Autodesk Inventor part; units mm, degrees
ref_plane "YZ Plane" through (0, 0, 0) normal (1, 0, 0) x (0, 1, 0)
ref_plane "XZ Plane" through (0, 0, 0) normal (0, 1, 0) x (-1, 0, 0)
ref_plane "XY Plane" through (0, 0, 0) normal (0, 0, 1) x (1, 0, 0)
sketch "Sketch2" plane through (0, 0, 0) normal (0, 1, 0) x (-1, 0, 0)
  line L0 (8.7236, 13.4517) -> (-1.2764, 13.4517)
  line L1 (-1.2764, 13.4517) -> (-1.2764, -3.0483)
  line L2 (-1.2764, -3.0483) -> (8.7236, -3.0483)
  line L3 (8.7236, -3.0483) -> (8.7236, 13.4517)
  point P0 (0, 0)
  dimension "d2" = 10
  dimension "d3" = 16.5
extrude "Extrusion1" add sketch "Sketch2" along normal blind 3
ref_plane "Work Plane1" through (-8.7236, 0, 6.9517) normal (0, 0, 1) x (1, 0, 0)
sketch "Sketch5" plane through (-8.7236, 0, 13.4517) normal (0, 0, 1) x (1, 0, 0)
  line L0 (0, 3) -> (10, 3)
  line L1 (-3, 0) -> (3, 0)
  line L2 (3, 0) -> (3, 6)
  line L3 (3, 6) -> (-3, 6)
  line L4 (-3, 6) -> (-3, 0)
  line L5 (0, 0) -> (10, 0)
  point P0 (8.7236, 0)
  dimension "d41" = 6
  dimension "d42" = 6
  dimension "d43" = 3
extrude "Extrusion4" cut sketch "Sketch5" against normal blind 6.5
sketch "Sketch6" plane through (-8.7236, 0, 6.9517) normal (0, 0, 1) x (1, 0, 0)
  circle A0 centre (0, 3) radius 3
  arc A1 (0, 0) -> (3, 3) centre (0, 3) ccw
  point P0 (8.7236, 0)
  point P1 (0, 0.5)
  dimension "d16" = 6
extrude "Extrusion5" add sketch "Sketch6" against normal blind 5
sketch "Sketch7" plane through (-8.7236, 0, 6.9517) normal (0, 0, 1) x (1, 0, 0)
  arc A0 (3, 3) -> (0, 0) centre (0, 3) ccw
  circle A1 centre (0, 3) radius 1.75
  line L0 (3, 0) -> (0, 0)
  line L1 (3, 3) -> (3, 0)
  point P0 (8.7236, 0)
  dimension "d20" = 3.5
extrude "Extrusion6" cut sketch "Sketch7" against normal up to next contours A1
sketch "Sketch9" plane through (0, 3, 0) normal (0, 1, 0) x (1, 0, 0)
  circle A0 centre (-3.2236, -9.4517) radius 1.75
  line L0 (1.2764, -13.4517) -> (1.2764, 3.0483)
  line L1 (-5.7236, -13.4517) -> (1.2764, -13.4517)
  point P0 (0, 0)
  dimension "d28" = 3.5
  dimension "d29" = 4.5
  dimension "d30" = 4
extrude "Extrusion8" cut sketch "Sketch9" against normal up to next
mirror "Mirror2" about plane through (1.2764, 0, -3.0483) normal (0, 0, -1)
sketch "Sketch10" plane through (0, 3, 0) normal (0, 1, 0) x (1, 0, 0)
  circle A0 centre (3.2764, -9.4517) radius 3
  circle A1 centre (3.2764, 15.5483) radius 3
  line L0 (1.2764, -13.4517) -> (1.2764, 19.5483)
  point P0 (0, 0)
  dimension "d33" = 6
  dimension "d34" = 6
  dimension "d35" = 2
  dimension "d36" = 4
  dimension "d37" = 4
  dimension "d40" = 2
extrude "Extrusion9" cut sketch "Sketch10" against normal through all
sketch "Sketch11" plane through (-8.7236, 0, 1.9517) normal (0, 0, -1) x (-1, 0, 0)
  line L0 (-3, 0) -> (-10, 0)
  line L1 (-3, 0) -> (3, 0)
  line L2 (3, 0) -> (3, 6)
  line L3 (3, 6) -> (-3, 6)
  line L4 (-3, 6) -> (-3, 0)
  point P0 (-8.7236, 0)
  dimension "d44" = 6
  dimension "d45" = 6
extrude "Extrusion10" cut sketch "Sketch11" along normal blind 10
equation "\"d33\" = d34"
equation "\"d37\" = d36"
equation "\"d40\" = d35"
properties part number "k2_hinge1_bot"
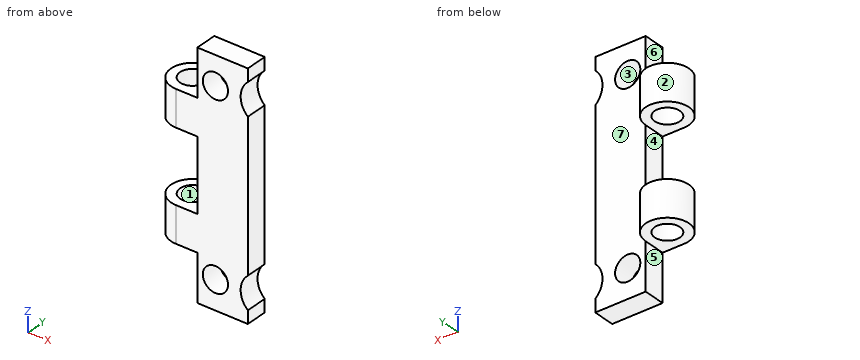
Geometry check sheet. Reference: the model listing, model coordinates, mm. Face numbers are marked on the shaded views. A direction names the side the tool comes from. Give positions to 0.01 mm unless a question says otherwise; leave off trailing zeros. Write each loop counter-clockwise with the first axis right and the second up, starting at its lowest first coordinate (ties: lowest second). Pieces come first, ordered by that corner, then holes.
1) Section check D-D, the plane z = -16. Record the boundary of the cut face in (x, y), and give its area (3 significant figures).
2) Gauge pin test, flat ends, axial feed: pin 1 (3 mm diameter, centred on x = -8.72, y = 3, fed in from -Z); pin 2 (1.5 mm diameter, centred on x = -10, z = -11, fed in from -Y); pin 3 (1.5 mm diameter, centred on y = 2, z = -16, fed in from -X); pin 4 (2 mm diameter, centred on x = -2, z = 5, fed in from +Y). Record the tip position at first contact, or that the pin passes through.
3) Section check A-A, the plane y = 2.45. Record the boundary of the cut face in (x, z), and give its area (3 significant figures).
4) Section check C-C, the plane y = 5.6. Record the boundary of the cut face in (x, z), and give its area (3 significant figures).
5) Release check for a two-part mould opening along Y. For the marked faces 1, 2 and 3 record: pulls with the +Y half, pulls with the -Y half, needs draft (parallel to the pull), parting line crosses it, or undercut.
6) Material ranges on L1, parallel to Z at x = -8.25, y = 4.95; L2, parallel to Z at x = -3.5, y = 1.75; L3, parallel to Z at x = -4.25, y = 0.35, recorded low to high.
7) Access from +Z, -Z, +X, -X, +Y, -Y to the whole of each face (thin tool, end or side, straight path). Record for the marked faces 4, 5, 6 and 7.
8) Section check B-B, the plane z = -11.5. Record the boundary of the cut face in (x, y), and give its area (3 significant figures).
Computed:
1. outline: (-5.72, 0) - (-4.91, 0) - (-4.91, 3) - (-5.72, 3) - close; (-1.53, 0) - (0.31, 0) - (0.31, 3) - (-1.53, 3) - close
1. area: 7.96 mm2
2. pin 1: passes through
2. pin 2: stops at y = 0.05
2. pin 3: stops at x = -5.72
2. pin 4: stops at y = 3
3. outline: (-11.67, -13.05) - (-10.38, -13.05) - (-10.38, -8.05) - (-11.67, -8.05) - close; (-11.67, 1.95) - (-10.38, 1.95) - (-10.38, 6.95) - (-11.67, 6.95) - close; (-7.06, -13.05) - (-5.72, -13.05) - (-5.72, -19.55) - (1.28, -19.55) - (1.28, -17.78) arc R3 cw to (1.28, -13.31) - (1.28, 7.22) arc R3 cw to (1.28, 11.69) - (1.28, 13.45) - (-5.72, 13.45) - (-5.72, 6.95) - (-7.06, 6.95) - (-7.06, 1.95) - (-5.72, 1.95) - (-5.72, -8.05) - (-7.06, -8.05) - close; hole circle Ø3.5 at (-3.22, -15.55); hole circle Ø3.5 at (-3.22, 9.45)
3. area: 232 mm2
4. outline: (-10.22, -13.05) - (-7.23, -13.05) - (-7.23, -8.05) - (-10.22, -8.05) - close; (-10.22, 1.95) - (-7.23, 1.95) - (-7.23, 6.95) - (-10.22, 6.95) - close
4. area: 29.9 mm2
5. face 1: undercut
5. face 2: parting line crosses it
5. face 3: needs draft
6. L1: z = -13.05 to -8.05, 1.95 to 6.95
6. L2: z = -19.55 to -17.28, -13.82 to 7.72, 11.18 to 13.45
6. L3: z = -19.55 to -16.97, -14.13 to 8.03, 10.87 to 13.45
7. face 4: -X, +Y, -Y
7. face 5: -Z, -X, +Y, -Y
7. face 6: +Z, -X, +Y, -Y
7. face 7: +Z, -Z, +X, +Y
8. outline: (-8.72, 0) - (1.28, 0) - (1.28, 3) - (-5.72, 3) arc R3 ccw (long way) to start; hole circle Ø3.5 at (-8.72, 3)
8. area: 41.6 mm2
